```python
from build123d import *

# Parameters (mm, degrees)
SKETCH_R           = 15
PAD_DEPTH          = 18
SKETCH001_W        = 2.525
SKETCH001_H        = 7
SKETCH002_R        = 4
POCKET_DEPTH       = 18.001
SKETCH003_W        = 6
SKETCH003_H        = 9
POCKET001_DEPTH    = 7
POLARPATTERN_COUNT = 40


with BuildPart() as part:
    # Sketch → Pad (new body)
    with BuildSketch(Plane.XY):
        Circle(SKETCH_R)
    extrude(amount=PAD_DEPTH)

    # Sketch001 → Groove (revolve, cut)
    with BuildSketch(Plane.XZ):
        with Locations((13.7375, 13.5)):
            Rectangle(SKETCH001_W, SKETCH001_H)
    revolve(axis=Axis((0, 0, 0), (0, 0, 1)), mode=Mode.SUBTRACT)

    # Sketch002 (on Face7 of Groove) → Pocket (cut, through all)
    with BuildSketch(Plane.XY.offset(18)):
        Circle(SKETCH002_R)
    extrude(amount=-POCKET_DEPTH, mode=Mode.SUBTRACT)

    # Sketch003 → Groove001 (revolve, cut)
    with BuildSketch(Plane.YZ):
        with Locations((12, 4.5)):
            Rectangle(SKETCH003_W, SKETCH003_H)
    revolve(axis=Axis((0, 0, 0), (0, 0, 1)), mode=Mode.SUBTRACT)

    # Sketch004 (on Face3 of Groove001) → Pocket001 (cut)
    with BuildSketch(Plane.XY.offset(10)):
        with BuildLine():
            ThreePointArc((12.46498, 0.4999), (11.975, 0), (12.46498, -0.4999))
            ThreePointArc((12.46498, -0.4999), (12.475, 0), (12.46498, 0.4999))
        make_face()
    pocket001 = extrude(amount=POCKET001_DEPTH, mode=Mode.SUBTRACT)

    # PolarPattern: Pocket001 ×40 about axis
    polarpattern_axis = Axis((0, 0, 10), (0, 0, 1))
    for i in range(1, POLARPATTERN_COUNT):
        add(pocket001.rotate(polarpattern_axis, i * 360 / POLARPATTERN_COUNT), mode=Mode.SUBTRACT)


solid = part.part
```
The model under review builds one solid part; all positions refer to its coordinate system, in mm. A direction names the side the tool comes from. Round coordinates to 2 decimals unless told otherwise and drop trailing zeros. Write each loop counter-clockwise with the first axis right and the second up, starting at its lowest first coordinate (ties: lowest second). Pieces come first, ordered by that corner, then holes.
(1) Insertion check: pin 1 (10 mm diameter, centred on y = -8, z = 14.5, fed in from +X); pin 2 (1.5 mm diameter, centred on y = 9, z = 6, fed in from -X); pin 3 (5 mm diameter, centred on y = -3.5, z = 5, fed in from -X). Each pin has a flat end and moves straight along its axis. Give the tip position at first contact, or say it passes through.
(2) We need section A-A on y = 0. Give the boundary of the cut face in (x, z) (3 decimals), and give its area (3 significant figures).
(3) We need section C-C on z = 4.25. Give the boundary of the cut face in (x, y), and give its area (3 significant figures).
(4) Mouldability with a two-part tool opening along Z and no side actions: class faces 1 (the flat face through (6.5, -6.5, 9)), 2 (the cylindrical face through (9.694, -7.03, 13.451)) as +Z half, -Z half, draft (parallel to the pull), parting line (faces both ways), or undercut.
(5) Wall thickness on L1, parallel to Z at x = -5, y = -13.5; L2, parallel to Z at x = -11.5, y = -2; L3, parallel to Y at x = -1, z = 8.5: over which ranges is each line inside the solid? List them lowest first.
(6) Machinability: for faces 3 (the cylindrical face through (-4.768, 11.528, 13.549)), 4 (the cylindrical face through (5.427, 10.675, 13.451)), 5 (the cylindrical face through (-2.92, -12.13, 13.55)), 6 (the cylindrical face through (4.78, 11.523, 13.549)), which of the approach directions +Z, -Z, +X, -X, +Y, -Y give a long, thin tool a straight path to every point of the face, cutting with its end or side? Answer none if there is none.
Findings below:
1. pin 1: stops at x = 14.54
1. pin 2: stops at x = -3.6
1. pin 3: stops at x = -8.94
2. outline: (-15, 9) - (-9, 9) - (-9, 0) - (-4, 0) - (-4, 18) - (-15, 18) - (-15, 17) - (-11.975, 17) - (-11.975, 10) - (-15, 10) - close; (4, 0) - (9, 0) - (9, 9) - (15, 9) - (15, 10) - (11.975, 10) - (11.975, 17) - (15, 17) - (15, 18) - (4, 18) - close
2. area: 246 mm2
3. outline: circle Ø18 at (0, 0); hole circle Ø8 at (0, 0)
3. area: 204 mm2
4. face 1: -Z half
4. face 2: undercut
5. L1: z = 9 to 10, 17 to 18
5. L2: z = 9 to 18
5. L3: y = -8.94 to -3.87, 3.87 to 8.94
6. face 3: -X, +Y
6. face 4: none
6. face 5: -X, -Y
6. face 6: +X, +Y
